from build123d import *

# Parameters (mm, degrees)
BOSS_EXTRUDE1_DEPTH = 4
BOSS_EXTRUDE2_DEPTH = 6
SKETCH4_R           = 2.25
CUT_EXTRUDE1_DEPTH  = 36.318797722
CUT_EXTRUDE2_REACH  = 28.63
SKETCH5_R           = 3.75
FILLET1_R           = 10
FILLET3_R           = 2


with BuildPart() as part:
    # Sketch2 → Boss-Extrude1 (new body)
    with BuildSketch(Plane(origin=(0, 0, 0), x_dir=(1, 0, 0), z_dir=(0, 1, 0))):
        Polygon((-32.718226242, 13.928959815), (-24.894958744, 23), (0, 23), (0, 13.928959815), (-19, 13.928959815), (-19, 0), (-25, 0), (-25, 7.27241908), align=None)
    extrude(amount=-BOSS_EXTRUDE1_DEPTH)

    # Sketch3 → Boss-Extrude2 (add)
    with BuildSketch(Plane(origin=(0, -4, 0), x_dir=(-1, 0, 0), z_dir=(0, 1, 0))):
        Polygon((25.757269356, -7.92552177), (32.718226242, -13.928959815), (24.894958744, -23), (20.894958744, -23), (20.894958744, -13.563347009), align=None)
    extrude(amount=-BOSS_EXTRUDE2_DEPTH)

    # Sketch4 → Cut-Extrude1 (cut, through all)
    with BuildSketch(Plane(origin=(-25.651402317, 0, -22.122907398), x_dir=(-0.653102689208867, 0, 0.7572693558755339), z_dir=(-0.7572693558755339, 0, -0.653102689208867))):
        with Locations((7.020387118, -5)):
            Circle(SKETCH4_R)
    extrude(amount=-CUT_EXTRUDE1_DEPTH, mode=Mode.SUBTRACT)

    # Cut-Extrude2: up to this plane
    cut_extrude2_end = Plane(origin=(-19, -4, -13.928959815), z_dir=(1, 0, 0))
    # Sketch5 → Cut-Extrude2 (cut, up to the surface)
    with BuildSketch(Plane(origin=(-18.690445431, 0, -16.119469352), x_dir=(0.6531026892088669, 0, -0.757269355875534), z_dir=(0.757269355875534, 0, 0.6531026892088669)), mode=Mode.PRIVATE) as cut_extrude2_sk1:
        with Locations((-7.020387118, -5)):
            Circle(SKETCH5_R)
    cut_extrude2_tool1 = split(extrude(cut_extrude2_sk1.sketch, amount=CUT_EXTRUDE2_REACH, mode=Mode.PRIVATE), bisect_by=cut_extrude2_end, keep=Keep.BOTH, mode=Mode.PRIVATE)
    add(cut_extrude2_tool1.solids().sort_by_distance((-23.275479, -5, -10.803145))[0], mode=Mode.SUBTRACT)

    # Fillet1
    fillet1_edges = [part.edges().sort_by_distance(p)[0] for p in [
        (-19, -2, -13.928959815),
    ]]
    fillet(fillet1_edges, radius=FILLET1_R)

    # Fillet3
    fillet3_edges = [part.edges().sort_by_distance(p)[0] for p in [
        (-20.894958744, -4, -18.281673505),
    ]]
    fillet(fillet3_edges, radius=FILLET3_R)


solid = part.part
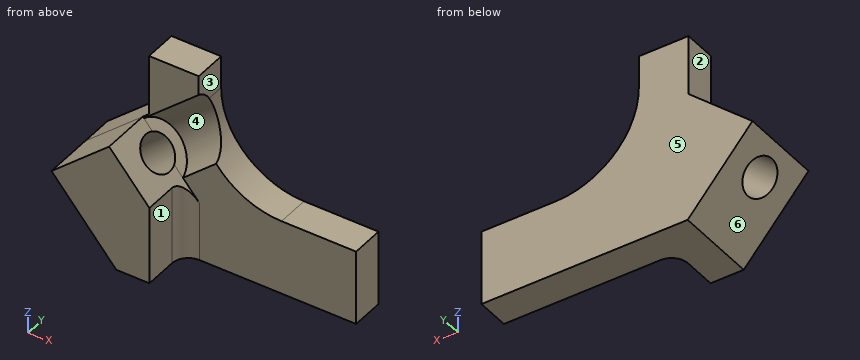
The listing builds one solid part. Answer for the finished solid, in the listing's coordinates (mm). Face numbers are marked on the shaded views. A direction names the side the tool comes from. Coordinates: 2 decimals unless noted, no trailing zeros. Order: outer loops, then holes, each group sorted by start corner. A loop starts at its lowest first (then second) coordinate and runs counter-clockwise, first axis right, second up.
Q1. Given P1, Ø2, axis at y = -2.5, z = -1, coming from the +X side; P2, Ø1.5, axis at y = -5.5, z = -13, coming from the +X side; P3, Ø5, axis at x = -7, z = -15.5, coming from the -Y side, each flat-ended and moving along its own axis, determine where each tip first touches the part or whether it passes through.
Q2. Consider line 1 (Y direction, x = -27, z = -13.75); line 2 (X direction, y = -3, z = -2); line 3 (Y direction, x = -8.5, z = -14). Determine where each line is inside the solid, lowest interval first.
Q3. A cutting plane is placed at B-B, the plane z = -19. Write down the section's boundary in (x, y).
Q4. Which of the six approach directions +Z, -Z, +X, -X, +Y, -Y give full straight-line access (tool end or side, diameter ignored) to the marked faces 1, 2 and 3?
Q5. A cutting plane is placed at A-A, the plane y = -3.25. Write down the section's boundary in (x, z).
Q6. A cutting plane is placed at C-C, the plane y = -8.25. Write down the section's boundary in (x, z), and give its area (3 significant figures).
Q7. A cutting plane is placed at D-D, the plane x = -4. Write down the section's boundary in (y, z), and give its area (3 significant figures).
Q8. For a pull along X with two mould halves and no side action, classify the marked faces 4, 5 and 6 as pulls with the +X half, pulls with the -X half, needs draft (parallel to the pull), parting line crosses it, or undercut.
Answers follow:
1. P1: stops at x = -19
1. P2: stops at x = -20.76
1. P3: stops at y = -4
2. line 1: y = -10 to -7.24, -2.76 to 0
2. line 2: x = -25 to -19
2. line 3: y = -4 to 0
3. outline: (-28.34, -10) - (-20.89, -10) - (-20.89, -6) arc R2 cw to (-18.89, -4) - (0, -4) - (0, 0) - (-28.34, 0) - close
4. face 1: +Z, -Z, +X, -Y
4. face 2: +Z, -X, +Y, -Y
4. face 3: +Z, +X, +Y, -Y
5. outline: (-32.72, -13.93) - (-31.16, -15.74) - (-24.2, -9.73) - (-25.44, -8.29) - (-19, -2.74) - (-19, 0) - (-25, 0) - (-25, -7.27) - close; (-29.31, -17.88) - (-24.89, -23) - (0, -23) - (0, -13.93) - (-9, -13.93) arc R10 cw to (-17.07, -9.83) - (-21.11, -13.31) - (-22.35, -11.87) - close
6. outline: (-32.72, -13.93) - (-24.89, -23) - (-20.89, -23) - (-20.89, -13.56) - (-25.76, -7.93) - close
6. area: 108 mm2
7. outline: (-4, -23) - (0, -23) - (0, -13.93) - (-4, -13.93) - close
7. area: 36.3 mm2
8. face 4: undercut
8. face 5: needs draft
8. face 6: pulls with the -X half
